The listing builds one solid part. Answer for the finished solid, in the listing's coordinates (mm). Coordinates: 2 decimals unless noted, no trailing zeros. Write each loop counter-clockwise with the first axis right and the second up, starting at its lowest first coordinate (ties: lowest second). Pieces come first, ordered by that corner, then holes. Notation, with made-up numbers: M 76,47 L 125,47 A16 cw 125,53 Z; hole C 20.5,-36 d4. An arc over 180 degrees is marked long. Answer as CSV lines item,"result".
```python
from build123d import *

# Parameters (mm, degrees)
F1_DEPTH = 5
F2_R     = 2
F3_R     = 2
F4_DEPTH = 25.4
F5_R     = 0.5


with BuildPart() as f1:
    # F0 (on Top) → F1 (new body)
    with BuildSketch(Plane.XY):
        Polygon((-30, -10), (16.9377624965, -10), (30, 10), (-16.9377624965, 10), align=None)
    extrude(amount=F1_DEPTH)

    # F2
    f2_edges = [f1.edges().sort_by_distance(p)[0] for p in [
        (6.531119, 10, 5),
        (-23.468881, 0, 5),
        (23.468881, 0, 5),
        (16.937762, -10, 2.5),
        (30, 10, 2.5),
        (23.468881, 0, 0),
        (6.531119, 10, 0),
        (-23.468881, 0, 0),
    ]]
    fillet(f2_edges, radius=F2_R)

    # F3 (on face) → F4 (cut)
    with BuildSketch(Plane.XY.offset(5)):
        with Locations((21.2572028662, 5.2613858901)):
            Circle(F3_R)
    extrude(amount=-F4_DEPTH, mode=Mode.SUBTRACT)

    # F5
    f5_edges = [f1.edges().sort_by_distance(p)[0] for p in [
        (19.257203, 5.261386, 5),
        (19.257203, 5.261386, 0),
    ]]
    fillet(f5_edges, radius=F5_R)


solid = f1.part
```
Q1. The mould has two halves that part along Y. Classify faces 1 (the flat face through (-7, -10, 2)), 2 (the cylindrical face through (4.38, 9.43, 4.4)), 3 (the cylindrical face through (23.105, 4.495, 2.528)): pulls with the +Y half, pulls with the -Y half, needs draft (parallel to the pull), parting line crosses it, or undercut.
Output:
face 1,"pulls with the -Y half"
face 2,"pulls with the +Y half"
face 3,"undercut"
Q2. Find section B-B (x = -7). Give the vertices of the cut face in (y, z), and give its area (3 significant figures).
Output:
outline,"M -10,0 L 8,0 A2 ccw 10,2 L 10,3 A2 ccw 8,5 L -10,5 Z"
area,"98.3 mm2"
Q3. Find section A-A (z = 3.75). Give the vertices of the cut face in (x, y) (3 decimals).
Output:
outline,"M -29.826,-10 L 15.855,-10 A2 ccw 16.997,-9.642 L 27.857,6.986 A1.854 ccw 26.305,9.854 L -16.859,9.854 Z; hole C 21.257,5.261 d4"
Q4. Straight lines are drawn through the part: line 1 (X direction, y = 3.5, z = 2.1); line 2 (X direction, y = -3.25, z = 0.6); line 3 (X direction, y = -8, z = 1.2). For each, find the intervals that lie inside material, in ascending order.
Output:
line 1,"-21.18 to 20.31, 22.2 to 25.75"
line 2,"-24.91 to 20.66"
line 3,"-28.49 to 18.04"
